Input: part model. Units: mm. Frame: model coordinates. Coordinates: 2 decimals unless noted, no trailing zeros. Order: outer loops, then holes, each group sorted by start corner. A loop starts at its lowest first (then second) coordinate and runs counter-clockwise, first axis right, second up. Notation, with made-up numbers: (40, 75.25) -> (47, 75.25) arc R18 ccw to (47, 108.25) -> close; hole circle Ø5 at (-27, 44.25). An arc over 180 degrees is marked (long way). One line per item, written item: value. Start each with the question number.
from build123d import *

# Parameters (mm, degrees)
SKETCH_1_R      = 4
EXTRUDE_1_DEPTH = 21


with BuildPart() as part:
    # 草图1 → 凸台-拉伸1 (new, symmetric)
    with BuildSketch(Plane(origin=(0, 0, 0), x_dir=(1, 0, 0), z_dir=(0, 1, 0))):
        with BuildLine():
            Line((-55, 10), (55, 10))
            ThreePointArc((55, 10), (58.535533906, 8.535533906), (60, 5))
            Line((60, 5), (60, -5))
            ThreePointArc((60, -5), (58.535533906, -8.535533906), (55, -10))
            Line((55, -10), (-55, -10))
            ThreePointArc((-55, -10), (-58.535533906, -8.535533906), (-60, -5))
            Line((-60, -5), (-60, 5))
            ThreePointArc((-60, 5), (-58.535533906, 8.535533906), (-55, 10))
        make_face()
        with Locations(Location((50, 0, 0), (0, 0, 90))):
            Circle(SKETCH_1_R, mode=Mode.SUBTRACT)
    extrude(amount=EXTRUDE_1_DEPTH, both=True)


solid = part.part
1) Mould query, pull axis X, two halves, no side actions, for faces 1 (the cylindrical face through (52.4, -0.3, 3.2)), 2 (the cylindrical face through (-59, 0, -8)), 3 (the flat face through (1, 21, 0)). Classes: +X half, -X half, draft (parallel to the pull), parting line (faces both ways), or undercut.
2) Ray query, line 1 along X through (y, z) = (-6.5, 0); line 2 along Z through (x, y) = (50, -1); line 3 along X through (y, z) = (-17, -5.5). Return the intervals inside material, ascending. Write a range as from..to.
3) Pin query (flat end, axial travel): pin 1 Ø2 at (y, z) = (9.5, 7.5) entering from -X. Return the tip coordinate at first contact, or that it passes through.
4) Section query A-A, the plane z = 0. Return the cut outline in (x, y), plus the area to 3 significant figures.
5) Section query C-C, the plane y = 16. Return the cut outline in (x, z), plus the area to 3 significant figures.
6) Section query B-B, the plane x = 50. Return the cut outline in (y, z).
Entries:
1. face 1: undercut
1. face 2: -X half
1. face 3: draft
2. line 1: x = -60..46, 54..60
2. line 2: z = -10..-4, 4..10
2. line 3: x = -59.97..59.97
3. pin 1: stops at x = -59.77
4. outline: (-60, -21) -> (46, -21) -> (46, 21) -> (-60, 21) -> close; (54, -21) -> (60, -21) -> (60, 21) -> (54, 21) -> close
4. area: 4,700 mm2
5. outline: (-60, -5) arc R5 ccw to (-55, -10) -> (55, -10) arc R5 ccw to (60, -5) -> (60, 5) arc R5 ccw to (55, 10) -> (-55, 10) arc R5 ccw to (-60, 5) -> close; hole circle Ø8 at (50, 0)
5. area: 2,330 mm2
6. outline: (-21, -10) -> (21, -10) -> (21, -4) -> (-21, -4) -> close; (-21, 4) -> (21, 4) -> (21, 10) -> (-21, 10) -> close
